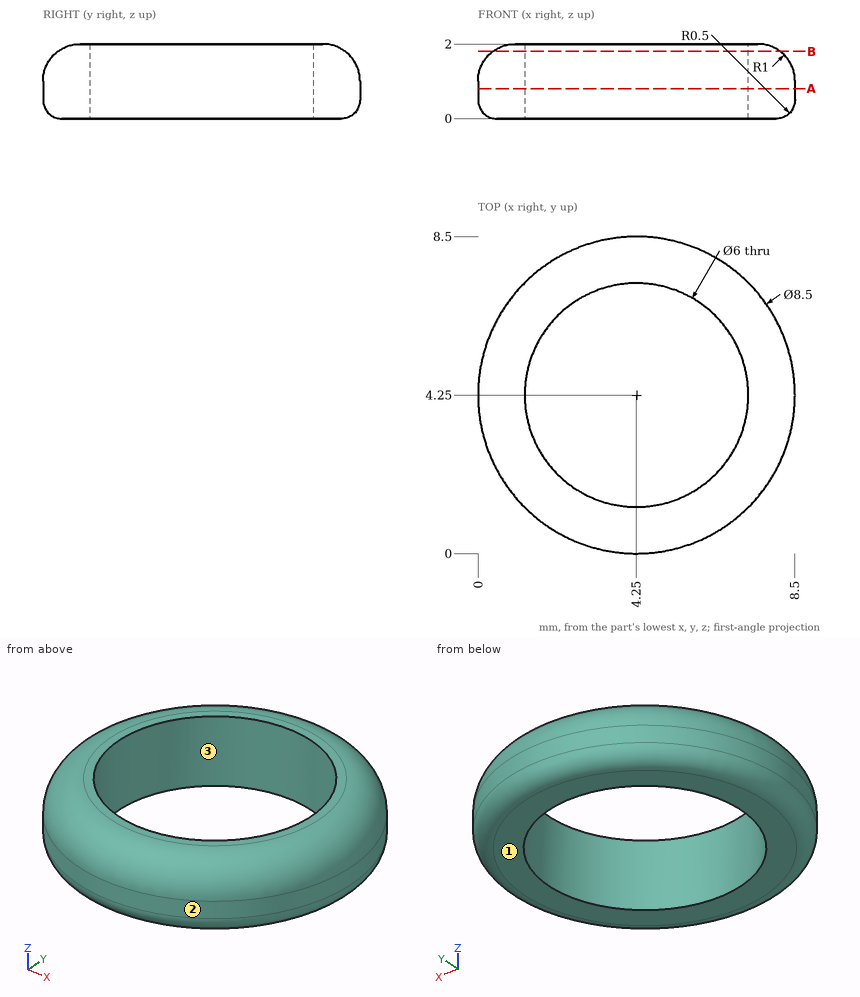
Input: dimensioned drawing with shaded views. Units: mm. Origin: part minimum x, y, z. Round coordinates to 2 decimals unless told otherwise and drop trailing zeros. Order: outer loops, then holes, each group sorted by start corner. A loop starts at its lowest first (then second) coordinate and runs counter-clockwise, first axis right, second up. Notation, with made-up numbers: (-12, 40.5) -> (19, 40.5) arc R34 ccw to (19, 78.5) -> close; hole circle Ø11 at (-23, -15). An arc over 180 degrees is marked (long way). One line per item, written item: value. Start each with the question number.
Q1. Material intervals for probe 1 along Y at (x, z) = (4.25, 0.8); probe 2 along Y at (x, z) = (4, 0.15); probe 3 along X at (y, z) = (2.75, 1.1), sorted ascending.
Q2. Pin query (flat end, axial travel): pin 1 (4 mm diameter, centred on x = 5.5, y = 2, fed in from +Z). Return the tip coordinate at first contact, or that it passes through.
Q3. Section query A-A (z = 0.8). Return the cut outline in (x, y), plus the area to 3 significant figures.
Q4. Draft query along X for the marked faces 1, 2 and 3. Return one class per face: pulls with the +X half, pulls with the -X half, needs draft (parallel to the pull), parting line crosses it, or undercut.
Q5. Section query B-B (z = 1.8). Return the cut outline in (x, y).
Findings below:
1. probe 1: 0 to 1.25, 7.25 to 8.5
1. probe 2: 0.15 to 1.26, 7.24 to 8.35
1. probe 3: 0.28 to 1.65, 6.85 to 8.22
2. pin 1: z = 2
3. outline: circle Ø8.5 at (4.25, 4.25); hole circle Ø6 at (4.25, 4.25)
3. area: 28.5 mm²
4. face 1: needs draft
4. face 2: parting line crosses it
4. face 3: undercut
5. outline: circle Ø7.7 at (4.25, 4.25); hole circle Ø6 at (4.25, 4.25)
